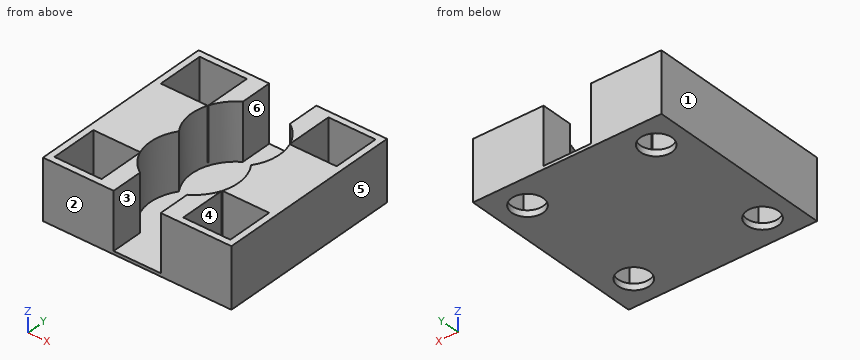
```python
from build123d import *

# Parameters (mm, degrees)
ESBO_O1_W                = 60
ESBO_O1_H                = 60
RESSALTO_EXTRUS_O2_DEPTH = 1
ESBO_O10_W               = 60
ESBO_O10_H               = 60
RESSALTO_EXTRUS_O5_DEPTH = 19
ESBO_O13_W               = 15
ESBO_O13_H               = 15
CORTE_EXTRUS_O7_DEPTH    = 17
ESBO_O14_R               = 5
CORTE_EXTRUS_O8_DEPTH    = 86.775773693
CORTE_EXTRUS_O9_START    = -18
ESBO_O15_R               = 4.5
CORTE_EXTRUS_O9_DEPTH    = 18


with BuildPart() as part:
    # Esboço1 → Ressalto-extrusão2 (new body)
    with BuildSketch(Plane.XY):
        with Locations((29.870134555, 28.412758376)):
            Rectangle(ESBO_O1_W, ESBO_O1_H)
    extrude(amount=RESSALTO_EXTRUS_O2_DEPTH)

    # Esboço10 → Ressalto-extrusão5 (add)
    with BuildSketch(Plane.XY):
        with Locations((29.870134555, 28.412758376)):
            Rectangle(ESBO_O10_W, ESBO_O10_H)
        with BuildLine():
            ThreePointArc((18.381009261, 28.412758376), (29.870134555, 6.412758376), (41.359259848, 28.412758376))
            ThreePointArc((41.359259848, 28.412758376), (29.870134555, 50.412758376), (18.381009261, 28.412758376))
        make_face(mode=Mode.SUBTRACT)
    extrude(amount=RESSALTO_EXTRUS_O5_DEPTH)

    # Esboço13 → Corte-extrusão7 (cut)
    with BuildSketch(Plane.XY.offset(19)):
        with Locations((9.370134555, 48.912758376)):
            Rectangle(ESBO_O13_W, ESBO_O13_H)
        with Locations((50.370134555, 48.912758376)):
            Rectangle(ESBO_O13_W, ESBO_O13_H)
        with Locations((9.370134555, 7.912758376)):
            Rectangle(ESBO_O13_W, ESBO_O13_H)
        with Locations((50.370134555, 7.912758376)):
            Rectangle(ESBO_O13_W, ESBO_O13_H)
    extrude(amount=-CORTE_EXTRUS_O7_DEPTH, mode=Mode.SUBTRACT)

    # Esboço14 → Corte-extrusão8 (cut, through all)
    with BuildSketch(Plane.XY.offset(19)):
        with Locations((9.370134555, 48.912758376)):
            Circle(ESBO_O14_R)
        with Locations((9.370134555, 7.912758376)):
            Circle(ESBO_O14_R)
        with Locations((50.370134555, 7.912758376)):
            Circle(ESBO_O14_R)
        with Locations((50.370134555, 48.912758376)):
            Circle(ESBO_O14_R)
    extrude(amount=-CORTE_EXTRUS_O8_DEPTH, mode=Mode.SUBTRACT)

    # Esboço15 → Corte-extrusão9 (cut)
    with BuildSketch(Plane.XY.offset(19).offset(CORTE_EXTRUS_O9_START)):
        with Locations((29.870134555, 28.412758376)):
            Circle(ESBO_O15_R)
        with BuildLine():
            Line((22.370134555, 8.591167958), (22.370134555, -1.587241624))
            Line((22.370134555, -1.587241624), (37.370134555, -1.587241624))
            Line((37.370134555, -1.587241624), (37.370134555, 8.591167958))
            ThreePointArc((37.370134555, 8.591167958), (29.870134555, 6.412758376), (22.370134555, 8.591167958))
        make_face()
        with BuildLine():
            Line((22.370134555, 58.412758376), (37.370134555, 58.412758376))
            Line((37.370134555, 58.412758376), (37.370134555, 48.234348794))
            ThreePointArc((37.370134555, 48.234348794), (29.870134555, 50.412758376), (22.370134555, 48.234348794))
            Line((22.370134555, 48.234348794), (22.370134555, 58.412758376))
        make_face()
    extrude(amount=CORTE_EXTRUS_O9_DEPTH, mode=Mode.SUBTRACT)


solid = part.part
```
Geometry check sheet. Reference: the model listing, model coordinates, mm. Face numbers are marked on the shaded views. A direction names the side the tool comes from. Coordinates: 2 decimals unless noted, no trailing zeros. Write each loop counter-clockwise with the first axis right and the second up, starting at its lowest first coordinate (ties: lowest second). Pieces come first, ordered by that corner, then holes. Notation, with made-up numbers: M 48,37 L 68,37 A18 ccw 68,53 Z; hole C 88,89.25 d3. An arc over 180 degrees is marked long. Use one line per item in the form item = value. Start each with the question number.
1) Section check D-D on y = 40.5. Enter the section's corners in (x, z).
2) Go/stop test with flat-tipped pins: pin 1 Ø7.5 at (x, y) = (8.5, 46) entering from +Z; pin 2 Ø14 at (x, y) = (32, 18.5) entering from +Z. Record where each tip stops, or that it passes through.
3) Set-up check for the marked faces 4, 5 and 6: record each of +Z, -Z, +X, -X, +Y, -Y from which the full face is reachable in a straight line by a thin tool's end or side.
4) Thickness scan on probe 1 along Y at (x, z) = (55, 8.5); probe 2 along X at (y, z) = (55.5, 17); probe 3 along X at (y, z) = (36.5, 8). Record the ranges inside material, lowest first. Write a range as from..to.
5) Section check A-A on y = 10.5. Enter the section's corners in (x, z), and give its area (3 significant figures).
6) Release check for a two-part mould opening along X. For the marked faces 1, 2 and 3 record: pulls with the +X half, pulls with the -X half, needs draft (parallel to the pull), parting line crosses it, or undercut.
7) Section check B-B on x = 48.5. Enter the section's corners in (y, z).
Responses:
q1.outline = M -0.13,0 L 59.87,0 L 59.87,19 L 43.26,19 L 43.26,1 L 16.48,1 L 16.48,19 L -0.13,19 Z
q2.pin_1 = 2
q2.pin_2 = 1
q3.face_4 = +Z
q3.face_5 = +Z, -Z, +X, +Y, -Y
q3.face_6 = +Z, +Y, -Y
q4.probe_1 = -1.59..0.41, 15.41..41.41, 56.41..58.41
q4.probe_2 = -0.13..1.87, 16.87..22.37, 37.37..42.87, 57.87..59.87
q4.probe_3 = -0.13..15.87, 43.87..59.87
q5.outline = M -0.13,0 L 5.09,0 L 5.09,2 L 1.87,2 L 1.87,19 L -0.13,19 Z; M 13.65,0 L 46.09,0 L 46.09,2 L 42.87,2 L 42.87,19 L 39.76,19 L 39.76,1 L 19.98,1 L 19.98,19 L 16.87,19 L 16.87,2 L 13.65,2 Z; M 54.65,0 L 59.87,0 L 59.87,19 L 57.87,19 L 57.87,2 L 54.65,2 Z
q5.area = 240 mm2
q6.face_1 = pulls with the -X half
q6.face_2 = needs draft
q6.face_3 = undercut
q7.outline = M -1.59,0 L 3.28,0 L 3.28,2 L 0.41,2 L 0.41,19 L -1.59,19 Z; M 12.55,0 L 44.28,0 L 44.28,2 L 41.41,2 L 41.41,19 L 15.41,19 L 15.41,2 L 12.55,2 Z; M 53.55,0 L 58.41,0 L 58.41,19 L 56.41,19 L 56.41,2 L 53.55,2 Z
